Check sheet for the modelled part. Datum: model origin and axes. Units: mm. Give positions to 0.01 mm unless a question says otherwise; leave off trailing zeros. Loops run counter-clockwise (first coordinate to the right, second up) from the corner with the lowest first, then second, coordinate; pieces in that order, holes last. Notation, with made-up numbers: (48.25, 10) -> (90.25, 10) arc R37 ccw to (90.25, 48) -> close; hole circle Ø9 at (39.25, 43.25). An arc over 180 degrees is marked (long way). Answer as CSV lines item,"result". Start each with the question number.
(1) Section check A-A on x = 0. Enter the section's corners in (y, z).
(2) Section check B-B on z = 25. Enter the section's corners in (x, y), plus the area to 3 significant figures.
(3) Gauge pin test, flat ends, axial feed: pin 1 Ø2.5 at (x, z) = (16.5, 0) entering from -Y; pin 2 Ø6 at (x, z) = (0, -30) entering from -Y; pin 3 Ø5 at (x, z) = (-16.5, 25) entering from -Y. Record the tip position at first contact, or that the pin passes through.
(4) Material ranges on line 1 (Z direction, x = -16.5, y = 4.15); line 2 (X direction, y = 3.75, z = 25); line 3 (Z direction, x = 0, y = 2.4), recorded low to high. Write a range as from..to.
from build123d import *

# Parameters (mm, degrees)
SKETCH_2_R                  = 2.2
EXTRUDE_1_DEPTH             = 5
SKETCH_3_R                  = 2
CUT_EXTRUDE_1_DEPTH         = 50
HOLE_WIZARD_M61_D           = 5
HOLE_WIZARD_M61_CSINK_D     = 7
HOLE_WIZARD_M61_CSINK_ANGLE = 90
HOLE_WIZARD_M41_D           = 4.5
HOLE_WIZARD_M41_CSINK_D     = 9.18
HOLE_WIZARD_M41_CSINK_ANGLE = 90


with BuildPart() as part:
    # Эскиз2 → Бобышка-Вытянуть1 (new body)
    with BuildSketch(Plane(origin=(0, 0, 0), x_dir=(1, 0, 0), z_dir=(0, 1, 0))):
        with BuildLine():
            Line((-16.5, -35), (16.5, -35))
            ThreePointArc((16.5, -35), (20.035533906, -33.535533906), (21.5, -30))
            Line((21.5, -30), (21.5, 30))
            ThreePointArc((21.5, 30), (20.035533906, 33.535533906), (16.5, 35))
            Line((16.5, 35), (-16.5, 35))
            ThreePointArc((-16.5, 35), (-20.035533906, 33.535533906), (-21.5, 30))
            Line((-21.5, 30), (-21.5, -30))
            ThreePointArc((-21.5, -30), (-20.035533906, -33.535533906), (-16.5, -35))
        make_face()
        with Locations(Location((-16.5, -25, 0), (0, 0, 270))):
            Circle(SKETCH_2_R, mode=Mode.SUBTRACT)
        with Locations(Location((-16.5, 0, 0), (0, 0, 270))):
            Circle(SKETCH_2_R, mode=Mode.SUBTRACT)
        with Locations(Location((-16.5, 25, 0), (0, 0, 270))):
            Circle(SKETCH_2_R, mode=Mode.SUBTRACT)
        with Locations(Location((16.5, 0, 0), (0, 0, 90))):
            Circle(SKETCH_2_R, mode=Mode.SUBTRACT)
        with Locations(Location((16.5, 25, 0), (0, 0, 90))):
            Circle(SKETCH_2_R, mode=Mode.SUBTRACT)
        with Locations(Location((16.5, -25, 0), (0, 0, 90))):
            Circle(SKETCH_2_R, mode=Mode.SUBTRACT)
    extrude(amount=EXTRUDE_1_DEPTH)

    # Эскиз3 → Вырез-Вытянуть1 (cut)
    with BuildSketch(Plane(origin=(0, 5, 0), x_dir=(1, 0, 0), z_dir=(0, 1, 0))):
        with Locations(Location((0, 30, 0), (0, 0, 270))):
            Circle(SKETCH_3_R)
        with Locations(Location((0, -30, 0), (0, 0, 270))):
            Circle(SKETCH_3_R)
    extrude(amount=-CUT_EXTRUDE_1_DEPTH, mode=Mode.SUBTRACT)

    # Отверстие обработанное метчиком M61 (through all)
    with Locations(Plane.XZ):
        with Locations((0, -30), (0, 30)):
            CounterSinkHole(HOLE_WIZARD_M61_D / 2, HOLE_WIZARD_M61_CSINK_D / 2, counter_sink_angle=HOLE_WIZARD_M61_CSINK_ANGLE)

    # Зенковка для винта с потайной головкой и внутренним шестигранником M41 (through all)
    with Locations(Plane.XZ):
        with Locations((16.5, -25), (16.5, 0), (16.5, 25), (-16.5, 25), (-16.5, 0), (-16.5, -25)):
            CounterSinkHole(HOLE_WIZARD_M41_D / 2, HOLE_WIZARD_M41_CSINK_D / 2, counter_sink_angle=HOLE_WIZARD_M41_CSINK_ANGLE)


solid = part.part
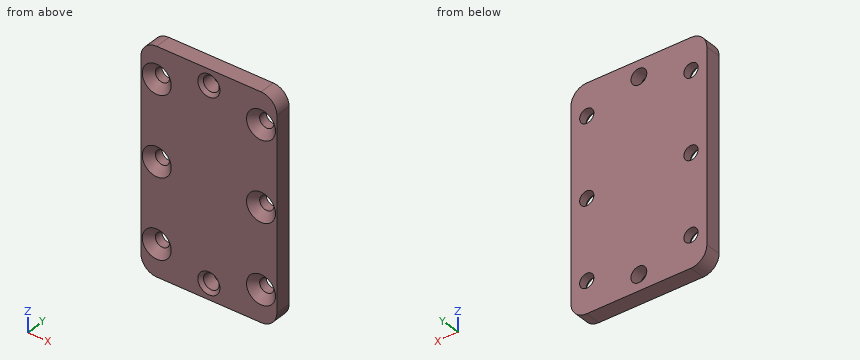
Working result:
1,outline,"(0, -35) -> (5, -35) -> (5, -32.5) -> (1, -32.5) -> (0, -33.5) -> close; (0, -26.5) -> (1, -27.5) -> (5, -27.5) -> (5, 27.5) -> (1, 27.5) -> (0, 26.5) -> close; (0, 33.5) -> (1, 32.5) -> (5, 32.5) -> (5, 35) -> (0, 35) -> close"
2,outline,"(-21.5, 0) -> (-21.09, 0) -> (-18.75, 2.34) -> (-18.75, 5) -> (-21.5, 5) -> close; (-14.25, 2.34) -> (-11.91, 0) -> (11.91, 0) -> (14.25, 2.34) -> (14.25, 5) -> (-14.25, 5) -> close; (18.75, 2.34) -> (21.09, 0) -> (21.5, 0) -> (21.5, 5) -> (18.75, 5) -> close"
2,area,"159 mm^2"
3,pin 1,"passes through"
3,pin 2,"stops at y = 0.5"
3,pin 3,"stops at y = 2.09"
4,line 1,"z = -35..-27.25, -22.75..-2.25, 2.25..22.75, 27.25..35"
4,line 2,"x = -21.5..-18.75, -14.25..14.25, 18.75..21.5"
4,line 3,"z = -35..-32.5, -27.5..27.5, 32.5..35"
